Geometry: see drawing. Coordinates: mm, zero at the bounding-box minimum. A direction names the side the tool comes from. Round coordinates to 2 decimals unless told otherwise and drop trailing zeros. Write each loop counter-clockwise with the first axis right and the second up, starting at its lowest first coordinate (ties: lowest second). Pieces come first, ordered by that corner, then holes. Notation, with made-up numbers: M 7.25,60 L 16.25,60 A24 cw 16.25,72 Z; hole C 82.5,63.5 d2. An arc over 180 degrees is marked long. Use one line per item in the form item = value. Start each with the question number.
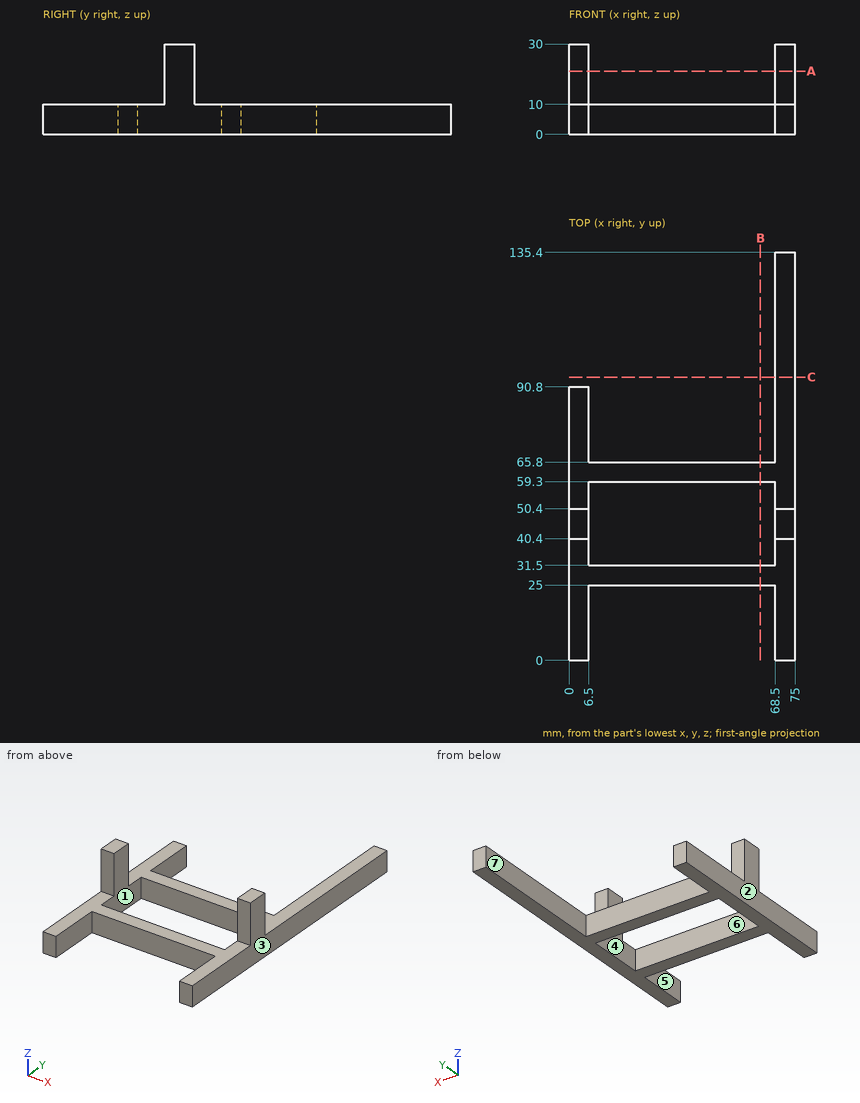
Item 1: Cut plane C-C (y = 94). Output: boundary loops of the cut face in (x, z).
Item 2: Cut plane B-B (x = 63.5). Output: boundary loops of the cut face in (y, z), plus the area to 3 significant figures.
Item 3: Cut plane A-A (z = 21). Output: boundary loops of the cut face in (x, y).
Item 4: Ray query, line 1 (Y direction, x = 39, z = 2.5); line 2 (Z direction, x = 6, y = 38); line 3 (Y direction, x = 70, z = 22.5). Return the intervals inside material, ascending. Write a range as from..to.
Item 5: Reachability of the marked faces 5, 6 and 7 from +Z, -Z, +X, -X, +Y, -Y: full face, straight path, thin tool, end or side. Return the list, or none.
Item 6: First-contact query: pin 1 (5 mm diameter, centred on x = 73, z = 21.5, fed in from +Y); pin 2 (11 mm diameter, centred on x = 22, z = 2.5, fed in from +Y); pin 3 (12 mm diameter, centred on x = 41.5, y = 27.5, fed in from +Z). Flat tips, straight axial feed; report the tip coordinate or a pass-through.
Item 7: Draft query along X for the marked faces 1, 2, 3 and 4. Return one class per face: +X half, -X half, draft (parallel to the pull), parting line (faces both ways), or undercut.
Final values:
q1.outline = M 68.5,0 L 75,0 L 75,10 L 68.5,10 Z
q2.outline = M 25,0 L 31.5,0 L 31.5,10 L 25,10 Z; M 59.3,0 L 65.8,0 L 65.8,10 L 59.3,10 Z
q2.area = 130 mm^2
q3.outline = M 0,40.4 L 6.5,40.4 L 6.5,50.4 L 0,50.4 Z; M 68.5,40.4 L 75,40.4 L 75,50.4 L 68.5,50.4 Z
q4.line_1 = 25..31.5, 59.3..65.8
q4.line_2 = 0..10
q4.line_3 = 40.4..50.4
q5.face_5 = +Z, -Z, -Y
q5.face_6 = +Z, -Z
q5.face_7 = +Z, -Z, +Y
q6.pin_1 = 50.4
q6.pin_2 = 65.8
q6.pin_3 = 10
q7.face_1 = undercut
q7.face_2 = -X half
q7.face_3 = +X half
q7.face_4 = undercut
